Verification items for the finished model (mm, model axes). Face numbers are marked on the shaded views. Round coordinates to 2 decimals unless told otherwise and drop trailing zeros. Write each loop counter-clockwise with the first axis right and the second up, starting at its lowest first coordinate (ties: lowest second). Pieces come first, ordered by that corner, then holes. Notation, with made-up numbers: M 23.25,21.5 L 77.25,21.5 A17 cw 77.25,41.5 Z; hole C 89,59.5 d10. An arc over 180 degrees is marked long. Answer in a Markdown table with one row per item. Add a question column.
1. Go/stop test with flat-tipped pins: pin 1 Ø12 at (x, y) = (-19.5, 41) entering from -Z; pin 2 Ø1.2 at (x, y) = (27, 43) entering from +Z; pin 3 Ø5 at (x, z) = (-14.5, -12) entering from +Y; pin 4 Ø6.5 at (x, z) = (15, 0) entering from -Y. Record where each tip stops, or that it passes through.
2. Material ranges on probe 1 along X at (y, z) = (0.5, 0); probe 2 along Z at (x, y) = (-7, 1); probe 3 along X at (y, z) = (37.5, -0.5) (3 decimals), recorded low to high.
3. Sectioned sample at C-C on x = 0. Record the cut outline in (y, z), plus the area to 3 significant figures.
4. Sectioned sample at A-A on x = -15. Record the cut outline in (y, z), plus the area to 3 significant figures.
5. Sectioned sample at B-B on z = -6. Record the cut outline in (x, y), plus the area to 3 significant figures.
6. Draft check along X on the marked faces 1 and 2. Enter one of: pulls with the +X half, pulls with the -X half, needs draft (parallel to the pull), parting line crosses it, or undercut.
7. Sectioned sample at D-D on y = 12. Record the cut outline in (x, z).
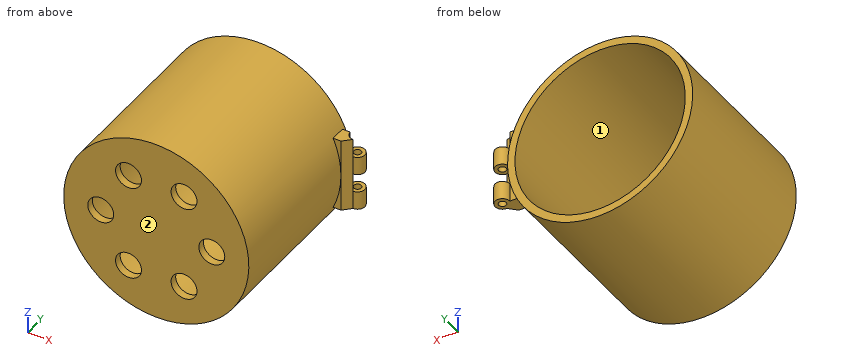
```python
from build123d import *

# Parameters (mm, degrees)
SKETCH1_R                = 25
BOSS_EXTRUDE1_DEPTH      = 45
SHELL1_T                 = -2
SKETCH2_R                = 3.5
CUT_EXTRUDE1_DEPTH       = 2
BOSS_EXTRUDE4_DEPTH      = 10
BOSS_EXTRUDE4_DEPTH_BACK = 10
BOSS_EXTRUDE6_REACH      = 74.395
SKETCH8_W                = 20
SKETCH8_H                = 4
CUT_EXTRUDE4_DEPTH       = 65.668384857
CUT_EXTRUDE4_DEPTH_BACK  = 65.668384857
SKETCH9_R                = 1
CUT_EXTRUDE5_START       = -5
SKETCH10_R               = 2
CUT_EXTRUDE5_DEPTH       = 5
LPATTERN2_COUNT          = 2
LPATTERN2_PITCH          = 10


with BuildPart() as part:
    # Sketch1 → Boss-Extrude1 (new body)
    with BuildSketch(Plane(origin=(0, 0, 0), x_dir=(1, 0, 0), z_dir=(0, 1, 0))):
        with Locations(Location((0, 0, 0), (0, 0, 90))):
            Circle(SKETCH1_R)
    extrude(amount=BOSS_EXTRUDE1_DEPTH)

    # Shell1
    shell1_openings = [part.faces().sort_by_distance(p)[0] for p in [
        (0, 45, 0),
    ]]
    offset(amount=SHELL1_T, openings=shell1_openings, kind=Kind.INTERSECTION)

    # Sketch2 → Cut-Extrude1 (cut)
    with BuildSketch(Plane(origin=(0, 2, 0), x_dir=(1, 0, 0), z_dir=(0, 1, 0))):
        with Locations(Location((15, 0, 0), (0, 0, 270))):
            Circle(SKETCH2_R)
        with Locations(Location((7.5, -12.990381057, 0), (0, 0, 270))):
            Circle(SKETCH2_R)
        with Locations(Location((-7.5, -12.990381057, 0), (0, 0, 270))):
            Circle(SKETCH2_R)
        with Locations(Location((-15, 0, 0), (0, 0, 270))):
            Circle(SKETCH2_R)
        with Locations(Location((-7.5, 12.990381057, 0), (0, 0, 270))):
            Circle(SKETCH2_R)
        with Locations(Location((7.5, 12.990381057, 0), (0, 0, 270))):
            Circle(SKETCH2_R)
    extrude(amount=-CUT_EXTRUDE1_DEPTH, mode=Mode.SUBTRACT)

    # Sketch8 → Boss-Extrude6 (add, up to next)
    with BuildSketch(Plane.ZY.offset(-25), mode=Mode.PRIVATE) as boss_extrude6_sk1:
        with Locations((0, 42)):
            Rectangle(SKETCH8_W, SKETCH8_H)
    boss_extrude6_tool1 = extrude(boss_extrude6_sk1.sketch, amount=BOSS_EXTRUDE6_REACH, mode=Mode.PRIVATE) - part.part


with BuildPart() as body_2:
    # Sketch3 → Boss-Extrude4 (new, two sides: drawn at the far end of the back side and taken through both)
    with BuildSketch(Plane.XY.offset(-BOSS_EXTRUDE4_DEPTH_BACK)):
        with BuildLine():
            Line((25, 44), (25, 40))
            Line((25, 40), (27, 42))
            ThreePointArc((27, 42), (28.414213562, 45.414213562), (25, 44))
        make_face()
    extrude(amount=BOSS_EXTRUDE4_DEPTH + BOSS_EXTRUDE4_DEPTH_BACK)


with BuildPart() as part_1:
    add(part.part)

    add(body_2.part)  # Boss-Extrude6 merges body 2
    add(boss_extrude6_tool1.solids().sort_by_distance((25, 42, 0))[0])
    add(boss_extrude6_tool1.solids().sort_by_distance((25, 42, 0))[1])

    # Sketch9 → Cut-Extrude4 (cut, two sides: drawn at the far end of the back side and taken through both)
    with BuildSketch(Plane.XY.offset(10).offset(-CUT_EXTRUDE4_DEPTH_BACK)):
        with Locations((27, 44)):
            Circle(SKETCH9_R)
    extrude(amount=CUT_EXTRUDE4_DEPTH + CUT_EXTRUDE4_DEPTH_BACK, mode=Mode.SUBTRACT)

    # Sketch10 → Cut-Extrude5 (cut)
    with BuildSketch(Plane.XY.offset(10).offset(CUT_EXTRUDE5_START)):
        with Locations((27, 44)):
            Circle(SKETCH10_R)
    cut_extrude5 = extrude(amount=CUT_EXTRUDE5_DEPTH, mode=Mode.SUBTRACT)

    # LPattern2: Cut-Extrude5 ×2
    with Locations(*[(0, 0, -i * LPATTERN2_PITCH) for i in range(1, LPATTERN2_COUNT)]):
        add(cut_extrude5, mode=Mode.SUBTRACT)


solid = part_1.part
```
Geometry check:
| question | item | result |
|---|---|---|
| 1 | pin 1 | stops at z = -21.04 |
| 1 | pin 2 | stops at z = 5 |
| 1 | pin 3 | stops at y = 2 |
| 1 | pin 4 | passes through |
| 2 | probe 1 | x = -25 to -18.5, -11.5 to 11.5, 18.5 to 25 |
| 2 | probe 2 | z = -24 to -16.45, -9.53 to 9.53, 16.45 to 24 |
| 2 | probe 3 | x = -24.995 to -22.995, 22.995 to 24.995 |
| 3 | outline | M 0,-25 L 45,-25 L 45,-23 L 2,-23 L 2,23 L 45,23 L 45,25 L 0,25 Z |
| 3 | area | 272 mm2 |
| 4 | outline | M 0,-20 L 45,-20 L 45,-17.44 L 2,-17.44 L 2,-3.5 L 0,-3.5 Z; M 0,3.5 L 2,3.5 L 2,17.44 L 45,17.44 L 45,20 L 0,20 Z |
| 4 | area | 287 mm2 |
| 5 | outline | M -24.27,0 L 24.27,0 L 24.27,40 L 25,40 L 27,42 A2 ccw long 25,44 L 24.27,44 L 24.27,45 L 22.2,45 L 22.2,2 L -22.2,2 L -22.2,45 L -24.27,45 Z; hole C 27,44 d2 |
| 5 | area | 290 mm2 |
| 6 | face 1 | undercut |
| 6 | face 2 | needs draft |
| 7 | outline | C 0,0 d50; hole C 0,0 d46 |
